Check sheet for the drawn part. Datum: minimum x, y, z corner. Units: mm. A direction names the side the tool comes from. Give positions to 0.01 mm unless a question says otherwise; leave off trailing zeros. Order: outer loops, then holes, each group sorted by start corner. A loop starts at its lowest first (then second) coordinate and runs counter-clockwise, first axis right, second up. Notation, with made-up numbers: M -1,78.25 L 40,78.25 A20 cw 40,99.25 Z; hole C -22,77.25 d10. An arc over 180 degrees is marked long. Answer as CSV lines item,"result". Start each with the question number.
Q1. Section check A-A, the plane y = 6.5. Record the boundary of the cut face in (x, z), then the cut area to 3 significant figures.
Q2. Thickness scan on line 1 (Y direction, x = 19, z = 18); line 2 (Y direction, x = 35, z = 33); line 3 (X direction, y = 31, z = 1). Record the ranges inside material, lowest first.
Q3. Section check D-D, the plane z = 33.5. Record the boundary of the cut face in (x, y).
Q4. Section check C-C, the plane z = 16.5. Count the separate pieces of the cut face and the enclosed holes in it, then the cut area to 3 significant figures.
Q5. Mould release check, pull along Y, two halves, no side actions. Record for the marked faces 1, 2 and 3: +Y half, -Y half, draft (parallel to the pull), parting line (faces both ways), or undercut.
Q6. Section check B-B, the plane x = 3. Record the boundary of the cut face in (y, z).
Q7. Set-up check for the marked faces 4 and 5: record each of +Z, -Z, +X, -X, +Y, -Y from which the full face is reachable in a straight line by a thin tool's end or side.
Q8. Go/stop test with flat-tipped pins: pin 1 (4 mm diameter, centred on y = 17, z = 29.5, fed in from +X); pin 2 (1 mm diameter, centred on y = 21, z = 5.5, fed in from +X) (1 decimal); pin 3 (1.5 mm diameter, centred on x = 35, y = 3, fed in from -Z); pin 4 (6.5 mm diameter, centred on x = 19, y = 31.5, fed in from -Z). Record where each tip stops, or that it passes through.
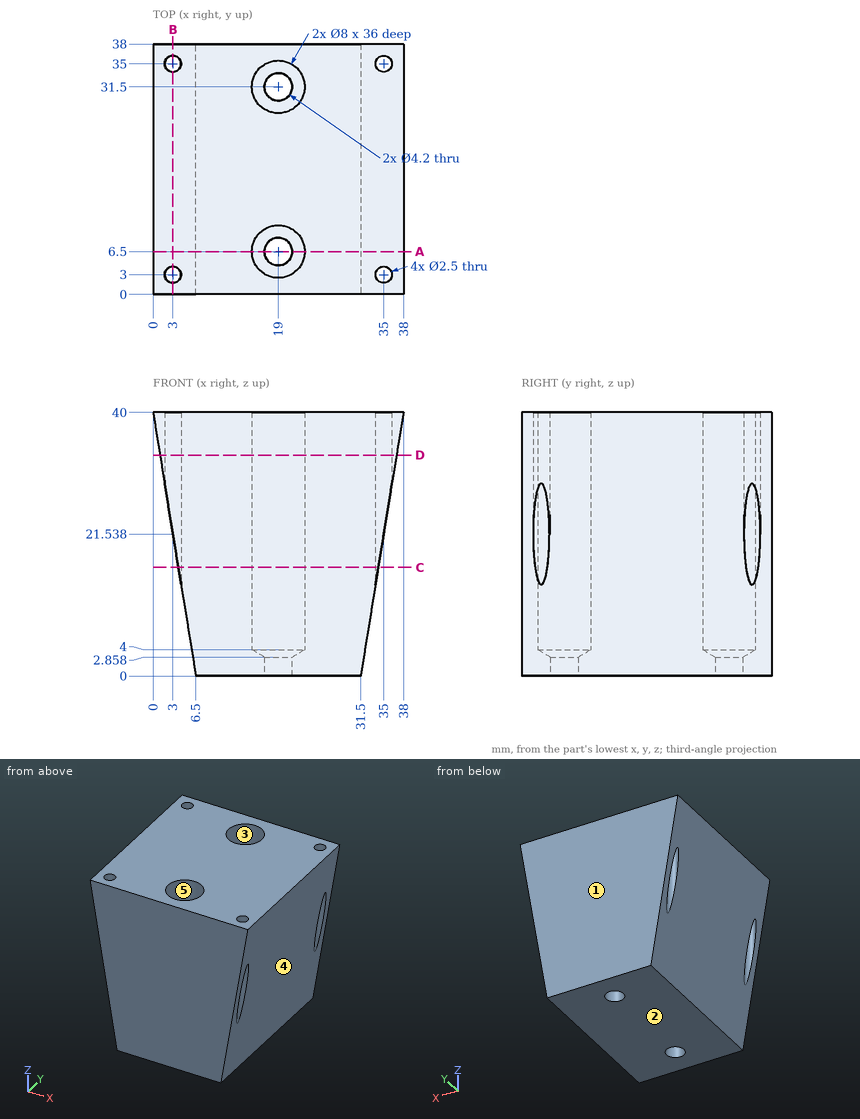
Answer block:
1,outline,"M 0,40 L 6.5,0 L 16.9,0 L 16.9,2.86 L 15,4 L 15,40 Z; M 21.1,0 L 31.5,0 L 38,40 L 23,40 L 23,4 L 21.1,2.86 Z"
1,area,"953 mm2"
2,line 1,"y = 0 to 2.5, 10.5 to 27.5, 35.5 to 38"
2,line 2,"y = 0 to 1.75, 4.25 to 33.75, 36.25 to 38"
2,line 3,"x = 6.34 to 16.96, 21.04 to 31.66"
3,outline,"M 1.06,0 L 36.94,0 L 36.94,38 L 1.06,38 Z; hole C 3,3 d2.5; hole C 3,35 d2.5; hole C 19,6.5 d8; hole C 19,31.5 d8; hole C 35,3 d2.5; hole C 35,35 d2.5"
4,separate pieces,"1"
4,enclosed holes,"2"
4,area,"1,050 mm2"
5,face 1,"+Y half"
5,face 2,"draft"
5,face 3,"undercut"
6,outline,"M 0,21.54 L 1.75,21.54 L 1.75,40 L 0,40 Z; M 4.25,21.54 L 33.75,21.54 L 33.75,40 L 4.25,40 Z; M 36.25,21.54 L 38,21.54 L 38,40 L 36.25,40 Z"
7,face 4,"-Z, +X, +Y, -Y"
7,face 5,"+Z"
8,pin 1,"stops at x = 36.62"
8,pin 2,"stops at x = 32.5"
8,pin 3,"passes through"
8,pin 4,"stops at z = 0"
